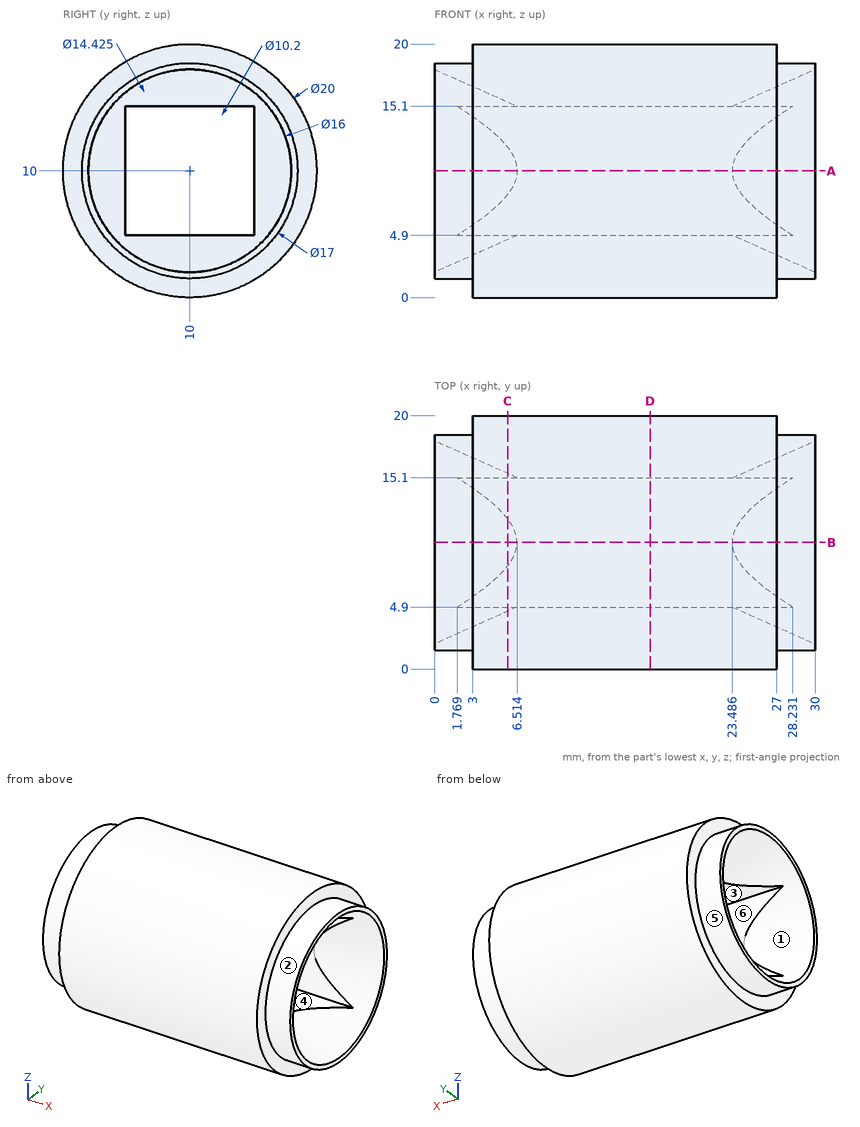
Print and shaded views of the part. All mm, measured from the part's lowest x, y and z. A direction names the side the tool comes from. Round coordinates to 2 decimals unless told otherwise and drop trailing zeros. Write each loop counter-clockwise with the first axis right and the second up, starting at its lowest first coordinate (ties: lowest second). Pieces come first, ordered by that corner, then holes. Notation, with made-up numbers: (88, 16) - (95, 16) arc R9 cw to (95, 31) - close; hole circle Ø1 at (-29.75, 39). An arc over 180 degrees is marked (long way). One line per item, written item: value.
(1) Two-plate mould, pull along Z, no slides. Class the marked faces 4, 5 and 6: pulls with the +Z half, pulls with the -Z half, needs draft (parallel to the pull), parting line crosses it, or undercut.
Values follow:
face 4: undercut
face 5: parting line crosses it
face 6: undercut
(2) 3-axis set-ups, long thin cutter, end or side, ignore diameter. For the marked faces 1, 2 and 3: which of +Z, -Z, +X, -X, +Y, -Y reach the whole face in a straight line?
Values follow:
face 1: -X
face 2: +X
face 3: +X, -X
(3) Wall check: probe 1 along Y at (x, z) = (18, 10.25); probe 2 along X at (y, z) = (4.75, 2.25). Give the ranges that are in metal, low to high.
Values follow:
probe 1: y = 0 to 4.9, 15.1 to 20
probe 2: x = 3 to 27
(4) Cut at D-D, the plane x = 17. Give the cut face in (y, z).
Values follow:
outline: circle Ø20 at (10, 10); hole (4.9, 4.9) - (15.1, 4.9) - (15.1, 15.1) - (4.9, 15.1) - close
(5) Drop flat-ended pins along their axis: P1, Ø3, axis at x = 24.5, z = 16, coming from the +Y side; P2, Ø4, axis at x = 12, z = 15.5, coming from the -Y side; P3, Ø1.5, axis at x = 12.5, z = 6.5, coming from the +Y side (1 decimal). Give the stop position or say it passes through.
Values follow:
P1: stops at y = 18.93
P2: stops at y = 0.63
P3: stops at y = 19.6
(6) Cut at A-A, the plane z = 10. Give the cut face in (x, y).
Values follow:
outline: (0, 1.5) - (3, 1.5) - (3, 0) - (27, 0) - (27, 1.5) - (30, 1.5) - (30, 2) - (23.49, 4.9) - (6.51, 4.9) - (0, 2) - close; (0, 18) - (6.51, 15.1) - (23.49, 15.1) - (30, 18) - (30, 18.5) - (27, 18.5) - (27, 20) - (3, 20) - (3, 18.5) - (0, 18.5) - close
(7) Cut at C-C, the plane x = 5.75. Give the cut face in (y, z), plus the area to 3 significant figures.
Values follow:
outline: circle Ø20 at (10, 10); hole (4.9, 4.9) - (8.11, 4.9) arc R5.44 ccw to (11.89, 4.9) - (15.1, 4.9) - (15.1, 8.11) arc R5.44 ccw to (15.1, 11.89) - (15.1, 15.1) - (11.89, 15.1) arc R5.44 ccw to (8.11, 15.1) - (4.9, 15.1) - (4.9, 11.89) arc R5.44 ccw to (4.9, 8.11) - close
area: 207 mm²
